Check sheet for the modelled part. Datum: model origin and axes. Units: mm. A direction names the side the tool comes from. Coordinates: 2 decimals unless noted, no trailing zeros. Loops run counter-clockwise (first coordinate to the right, second up) from the corner with the lowest first, then second, coordinate; pieces in that order, holes last.
Autodesk Inventor part; units mm, degrees
ref_plane "YZ Plane" through (0, 0, 0) normal (1, 0, 0) x (0, 1, 0)
ref_plane "XZ Plane" through (0, 0, 0) normal (0, 1, 0) x (-1, 0, 0)
ref_plane "XY Plane" through (0, 0, 0) normal (0, 0, 1) x (1, 0, 0)
sketch "Sketch6" plane through (0, 0, 0) normal (0, 1, 0) x (-1, 0, 0)
  line L0 (4.5, -6.1) -> (60.5, -6.1)
  line L1 (60.5, -6.1) -> (60.5, -90.9)
  line L2 (4.5, -90.9) -> (4.5, -6.1)
  line L3 (65.1201, -97) -> (0, -97)
  line L4 (0, -97) -> (0, 0)
  line L5 (0, 0) -> (65.1201, 0)
  line L6 (65.1201, 0) -> (65.1201, -97)
  line L7 (60.5, -90.9) -> (4.5, -90.9)
  line L8 (102.5, -48.5) -> (-37.5, -48.5)
  line L9 (32.5, -118.5) -> (32.5, 21.5)
  circle A0 centre (32.5, -48.5) radius 70
  line L10 (102.5, -48.5) -> (67.5, -109.1218)
  line L11 (67.5, -109.1218) -> (-2.5, -109.1218)
  line L12 (-2.5, -109.1218) -> (-37.5, -48.5)
  line L13 (-37.5, -48.5) -> (-2.5, 12.1218)
  line L14 (-2.5, 12.1218) -> (67.5, 12.1218)
  line L15 (67.5, 12.1218) -> (102.5, -48.5)
  line L16 (32.5, 12.1218) -> (85, -18.1891)
  line L17 (85, -18.1891) -> (85, -78.8109)
  line L18 (85, -78.8109) -> (32.5, -109.1218)
  line L19 (32.5, -109.1218) -> (-20, -78.8109)
  line L20 (-20, -78.8109) -> (-20, -18.1891)
  line L21 (-20, -18.1891) -> (32.5, 12.1218)
  line L22 (32.5, 12.1218) -> (47.5, 12.1218)
  line L23 (47.5, 12.1218) -> (47.5, 5.6218)
  line L24 (47.5, 5.6218) -> (17.5, 5.6218)
  line L25 (17.5, 5.6218) -> (17.5, 12.1218)
  line L26 (47.5, 5.6218) -> (56.6924, 5.6218) construction
  line L27 (17.5, 8.8718) -> (20, 8.8718)
  line L28 (47.5, 8.8718) -> (45, 8.8718)
  line L29 (45, 8.8718) -> (45, 10.1218)
  line L30 (45, 10.1218) -> (20, 10.1218)
  line L31 (20, 10.1218) -> (20, 7.6218)
  line L32 (20, 7.6218) -> (45, 7.6218)
  line L33 (45, 7.6218) -> (45, 10.1218)
  line L34 (67.5, 12.1218) -> (32.5, -48.5)
  line L35 (32.5, -48.5) -> (67.5, -109.1218)
  line L36 (47.5, 5.6218) -> (56.6924, 5.6218)
  line L37 (17.5, 5.6218) -> (11, 5.6218)
  line L38 (17.5, 12.1218) -> (11, 5.6218)
  line L39 (17.5, 12.1218) -> (26.6924, 12.1218) construction
  line L40 (47.5, 12.1218) -> (54, 5.6218)
  line L41 (85, -18.1891) -> (77.5, -5.1987)
  line L42 (77.5, -5.1987) -> (71.8708, -8.4487)
  line L43 (71.8708, -8.4487) -> (86.8708, -34.4295)
  line L44 (86.8708, -34.4295) -> (92.5, -31.1795)
  line L45 (71.8708, -8.4487) -> (67.2746, -0.4879) construction
  line L46 (89.6854, -32.8045) -> (88.4354, -30.6394)
  line L47 (74.6854, -6.8237) -> (75.9354, -8.9888)
  line L48 (75.9354, -8.9888) -> (77.0179, -8.3638)
  line L49 (77.0179, -8.3638) -> (89.5179, -30.0144)
  line L50 (89.5179, -30.0144) -> (87.3529, -31.2644)
  line L51 (87.3529, -31.2644) -> (74.8529, -9.6138)
  line L52 (74.8529, -9.6138) -> (77.0179, -8.3638)
  line L53 (71.8708, -8.4487) -> (67.2746, -0.4879)
  line L54 (86.8708, -34.4295) -> (90.1208, -40.0587)
  line L55 (92.5, -31.1795) -> (90.1208, -40.0587)
  line L56 (92.5, -31.1795) -> (87.9038, -23.2187) construction
  line L57 (77.5, -5.1987) -> (68.6208, -2.8196)
  line L58 (71.8708, -88.5513) -> (67.2746, -96.5121) construction
  line L59 (74.6854, -90.1763) -> (75.9354, -88.0112)
  line L60 (74.8529, -87.3862) -> (77.0179, -88.6362)
  line L61 (77.5, -91.8013) -> (71.8708, -88.5513)
  line L62 (77.5, -91.8013) -> (68.6208, -94.1804)
  line L63 (71.8708, -88.5513) -> (67.2746, -96.5121)
  line L64 (77.0179, -88.6362) -> (89.5179, -66.9856)
  line L65 (87.3529, -65.7356) -> (74.8529, -87.3862)
  line L66 (71.8708, -88.5513) -> (86.8708, -62.5705)
  line L67 (89.5179, -66.9856) -> (87.3529, -65.7356)
  line L68 (89.6854, -64.1955) -> (88.4354, -66.3606)
  line L69 (86.8708, -62.5705) -> (92.5, -65.8205)
  line L70 (86.8708, -62.5705) -> (90.1208, -56.9413)
  line L71 (92.5, -65.8205) -> (90.1208, -56.9413)
  line L72 (94.9944, -48.5) -> (63.7472, -102.6218)
  line L73 (63.7472, -102.6218) -> (1.2528, -102.6218)
  line L74 (1.2528, -102.6218) -> (-29.9944, -48.5)
  line L75 (-29.9944, -48.5) -> (1.2528, 5.6218)
  line L76 (1.2528, 5.6218) -> (63.7472, 5.6218)
  line L77 (63.7472, 5.6218) -> (94.9944, -48.5)
  line L78 (74.8529, -87.3862) -> (73.1208, -86.3862)
  line L79 (87.3529, -65.7356) -> (85.6208, -64.7356)
  line L80 (87.3529, -31.2644) -> (85.6208, -32.2644)
  line L81 (74.8529, -9.6138) -> (73.1208, -10.6138)
  line L82 (45, 7.6218) -> (45, 5.6218)
  line L83 (20, 7.6218) -> (20, 5.6218)
  line L84 (60.5, -90.9) -> (4.4985, -90.9)
  line L85 (4.4985, -90.9) -> (4.4985, -97)
  line L86 (4.4985, -97) -> (60.5, -97)
  line L87 (60.5, -97) -> (60.5, -90.9)
  line L88 (60.5, -6.1) -> (4.4985, -6.1)
  line L89 (4.4985, -6.1) -> (4.4985, 0)
  line L90 (4.4985, 0) -> (60.5, 0)
  line L91 (60.5, 0) -> (60.5, -6.1)
  dimension "d44" = 97
  dimension "d77" = 140
  dimension "d87" = 15
  dimension "d88" = 6.5
  dimension "d89" = 30
  dimension "d91" = 2.5
  dimension "d92" = 2.5
  dimension "d95" = 1.25
  dimension "d96" = 25
  dimension "d97" = 2.5
  dimension "d98" = 25
  dimension "d99" = 135
  dimension "d100" = 0
extrude "Fronte" add sketch "Sketch6" along normal blind 2 contours L89 L21 L5 L9 L0 | L2 L8 L4 L21 L89 | L9 L5 L16 L34 L0 | L2 L85 L19 L4 L8 | L89 L5 L21 | L21 L4 L5 L89 | L34 L16 L91 L0 | L9 L24 L16 L5 | L5 L21 L24 L9 | L7 L9 L3 L19 L85 | L8 L20 L75 L21 L4 | L4 L19 L74 L20 L8 | L21 L75 L76 L37 L24 L5 L4 | L91 L16 L6 L8 L1 | L34 L91 L16 | L16 L5 L34 | L8 L6 L18 L87 L1 | L7 L35 L18 L3 L9 | L7 L87 L18 L35 | L16 L24 L36 L76 L34 L5 | L24 L21 L32 L9 | L9 L32 L16 L24 | L85 L3 L4 L19 | L19 L3 L85 | L4 L3 L19 L73 L74 | L20 L74 L8 | L8 L75 L20 | L75 L20 L21 | L21 L13 L14 L38 L76 L75 | L24 L83 L32 L21 | L91 L5 L6 L16 | L34 L77 L53 L43 L16 L6 L5 | L8 L17 L66 L18 L6 | L6 L16 L43 L17 L8 | L9 L73 L19 L3 | L3 L18 L73 L9 | L35 L3 L18 | L18 L87 L35 | L16 L32 L82 L24 | L32 L21 L30 L9 | L9 L30 L16 L32 | L74 L73 L19 L11 L12 | L19 L20 L74 | L74 L20 L12 L8 | L8 L13 L20 L75 | L32 L31 L30 L21 | L24 L25 L27 L31 L83 | L76 L36 L40 L14 L34 | L34 L15 L57 L53 L77 | L18 L6 L3 L87 | L18 L66 L63 L72 L35 L3 L6 | L17 L43 L54 L77 L8 | L8 L72 L70 L66 L17 | L3 L35 L73 L18 | L73 L18 L9 | L9 L19 L73 | L16 L30 L29 L33 L32 | L82 L33 L28 L23 L24 | L30 L21 L9 | L9 L16 L30 | L38 L25 L37 | L30 L31 L27 L25 L14 L21 | L43 L81 L51 L16 | L16 L51 L17 L43 | L66 L17 L65 L18 | L18 L65 L78 L66 | L77 L55 L15 L8 | L8 L10 L71 L72 | L17 L51 L80 L43 | L66 L79 L65 L17 | L73 L35 L11 L18 | L72 L63 L62 L10 L35 | L16 L14 L23 L28 L29 L30 | L23 L40 L36 | L51 L52 L48 L49 L16 | L16 L49 L17 L51 | L43 L42 L47 L52 L81 | L15 L16 L49 L48 L47 L42 | L42 L53 L57 | L65 L17 L64 L18 | L18 L64 L60 L65 | L78 L60 L59 L61 L66 | L71 L69 L70 | L54 L44 L55 | L17 L49 L50 L51 | L80 L50 L46 L44 L43 | L65 L67 L64 L17 | L66 L69 L68 L67 L79 | L16 L17 L49 | L10 L17 L64 L67 L68 L69 | L44 L46 L50 L49 L17 L15 | L64 L17 L18 | L18 L10 L61 L59 L60 L64 | L61 L62 L63
extrude "Esterno" add sketch "Sketch6" against normal blind 25 contours L75 L20 L21 | L21 L13 L14 L38 L76 L75 | L74 L73 L19 L11 L12 | L19 L20 L74 | L74 L20 L12 L8 | L8 L13 L20 L75 | L76 L36 L40 L14 L34 | L34 L15 L57 L53 L77 | L73 L18 L9 | L9 L19 L73 | L77 L55 L15 L8 | L8 L10 L71 L72 | L73 L35 L11 L18 | L72 L63 L62 L10 L35
extrude "Strip" add sketch "Sketch6" against normal blind 10 contours L24 L21 L32 L9 | L9 L32 L16 L24 | L24 L83 L32 L21 | L16 L32 L82 L24 | L24 L25 L27 L31 L83 | L82 L33 L28 L23 L24 | L30 L21 L9 | L9 L16 L30 | L38 L25 L37 | L30 L31 L27 L25 L14 L21 | L43 L81 L51 L16 | L16 L51 L17 L43 | L66 L17 L65 L18 | L18 L65 L78 L66 | L17 L51 L80 L43 | L66 L79 L65 L17 | L16 L14 L23 L28 L29 L30 | L23 L40 L36 | L43 L42 L47 L52 L81 | L15 L16 L49 L48 L47 L42 | L42 L53 L57 | L78 L60 L59 L61 L66 | L71 L69 L70 | L54 L44 L55 | L80 L50 L46 L44 L43 | L66 L69 L68 L67 L79 | L16 L17 L49 | L10 L17 L64 L67 L68 L69 | L44 L46 L50 L49 L17 L15 | L64 L17 L18 | L18 L10 L61 L59 L60 L64 | L61 L62 L63
sketch "Sketch7" plane through (0, -25, 0) normal (0, -1, 0) x (1, 0, 0)
  line L0 (-17.5, 12.1218) -> (-17.5, -109.1218)
  line L1 (-67.5, -109.1218) -> (2.5, -109.1218)
  line L2 (-47.5, 12.1218) -> (-67.5, 12.1218)
  line L3 (-47.5, 12.1218) -> (-47.5, -109.1218)
  line L4 (-77.5, -91.8013) -> (-67.5, -109.1218)
  line L5 (-77.5, -91.8013) -> (27.5, -31.1795)
  line L6 (2.5, 12.1218) -> (37.5, -48.5)
  line L7 (-92.5, -65.8205) -> (-90.1208, -56.9413)
  line L8 (-92.5, -65.8205) -> (12.5, -5.1987)
  line L9 (-77.5, -5.1987) -> (27.5, -65.8205)
  line L10 (37.5, -48.5) -> (2.5, -109.1218)
  line L11 (-92.5, -31.1795) -> (11.423, -93.6666)
  line L12 (27.5, -31.1795) -> (12.5, -5.1987)
  line L13 (27.5, -65.8205) -> (11.423, -93.6666)
  line L14 (-1.2528, -102.6218) -> (29.9944, -48.5)
  line L15 (5.8516, -90.3166) -> (21.8708, -62.5705)
  line L16 (-47.5, -109.1218) -> (-17.5, -109.1218)
  line L17 (-17.5, -109.1218) -> (-17.5, -102.6218)
  line L18 (-17.5, -102.6218) -> (-47.5, -102.6218)
  line L19 (-47.5, -102.6218) -> (-47.5, -109.1218)
  line L20 (5.5339, -9.2206) -> (17.5, -36.953)
  point P0 (0, 0)
  point P1 (6.9325, -8.4131)
  point P2 (21.9325, -34.3939)
extrude "Passacavi" cut sketch "Sketch7" against normal blind 3 contours L0 L1 L3 L18 | L14 L9 L10 L11 | L20 L8 L6 L5
extrude "ScavoStrip" cut sketch "Sketch6" against normal blind 5 contours L24 L21 L32 L9 | L9 L32 L16 L24 | L24 L83 L32 L21 | L16 L32 L82 L24 | L43 L81 L51 L16 | L16 L51 L17 L43 | L66 L17 L65 L18 | L18 L65 L78 L66 | L17 L51 L80 L43 | L66 L79 L65 L17
extrude "ScreenDis1" add sketch "Sketch6" against normal blind 1 contours L7 L9 L3 L19 L85 | L7 L35 L18 L3 L9 | L7 L87 L18 L35 | L19 L3 L85 | L35 L3 L18 | L18 L87 L35
extrude "ScreenDist1.8" add sketch "Sketch6" against normal blind 1.8 contours L89 L21 L5 L9 L0 | L9 L5 L16 L34 L0 | L89 L5 L21 | L34 L16 L91 L0 | L34 L91 L16 | L16 L5 L34
properties part number "Hexagone" material "Wood (Cherry)"
1) Section check B-B on z = -80. Enter the section's corners in (x, y).
Answer sheet:
outline: (-84.31, -10) - (-82, -10) - (-82, 0) - (-60.5, 0) - (-60.5, 2) - (-84.31, 2) - close; (-79.12, -10) - (-76.81, -10) - (-76.81, -5) - (-79.12, -5) - close; (-4.5, 0) - (11.81, 0) - (11.81, -22) - (19.31, -22) - (19.31, 2) - (-4.5, 2) - close
2) Depth check by flat-ended pin: pin 1 (1.8 mm diameter, centred on x = -45, z = -2, fed in from -Y); pin 2 (1.4 mm diameter, centred on y = -0.5, z = -2, fed in from -X); pin 3 (0.6 mm diameter, centred on y = 1.5, z = -33, fed in from +X). Enter the tip coordinate at first touch or a pass-through.
Answer sheet:
pin 1: stops at y = -1.8
pin 2: stops at x = -76.06
pin 3: stops at x = 28.72
3) Scan lines: line 1 (Z direction, x = -26, y = -7); line 2 (Z direction, x = -12.5, y = -6.25); line 3 (Z direction, x = -42, y = -2.75). Record each from-to range of solid material in increasing order.
Answer sheet:
line 1: z = -109.12 to -102.62, 5.62 to 7.62, 10.12 to 12.12
line 2: z = -109.12 to -102.62, 5.62 to 12.12
line 3: z = -109.12 to -102.62, 10.12 to 12.12
4) Section check C-C on x = -57. Enter the section's corners in (y, z).
Answer sheet:
outline: (-25, -109.12) - (2, -109.12) - (2, -90.9) - (-1, -90.9) - (-1, -97) - (0, -97) - (0, -102.62) - (-25, -102.62) - close; (-25, 5.62) - (0, 5.62) - (0, 0) - (-1.8, 0) - (-1.8, -6.1) - (2, -6.1) - (2, 12.12) - (-25, 12.12) - close
5) Section check D-D on z = -36. Enter the section's corners in (x, y), plus the area to 3 significant figures.
Answer sheet:
outline: (-95.28, -25) - (-91.21, -25) - (-91.21, -10) - (-87.78, -10) - (-87.78, 0) - (-60.5, 0) - (-60.5, 2) - (-95.28, 2) - close; (-4.5, 0) - (22.78, 0) - (22.78, -25) - (30.28, -25) - (30.28, 2) - (-4.5, 2) - close
area: 463 mm2
6) Mould release check, pull along Z, two halves, no side actions. Record for faces 1 (the flat face through (24.646, -23.521, -32.827)), 2 (the flat face through (-73.123, -17.395, -4.026)), 3 (the flat face through (-91.327, -17.395, -61.443)): +Z half, -Z half, draft (parallel to the pull), parting line (faces both ways), or undercut.
Answer sheet:
face 1: +Z half
face 2: undercut
face 3: -Z half
7) Set-up check for faces 4 (the flat face through (-33, -22, -106)), 5 (the flat face through (-32, 0, -6.1)), 6 (the flat face through (-80.5, -10, -20)): record each of +Z, -Z, +X, -X, +Y, -Y from which the full face is reachable in a straight line by a thin tool's end or side.
Answer sheet:
face 4: +Z, -Z, -Y
face 5: +Y, -Y
face 6: -Y
8) Section check A-A on x = -27. Enter the section's corners in (y, z).
Answer sheet:
outline: (-22, -109.12) - (2, -109.12) - (2, -90.9) - (-1, -90.9) - (-1, -97) - (0, -97) - (0, -102.62) - (-22, -102.62) - close; (-10, 5.62) - (-5, 5.62) - (-5, 7.62) - (-10, 7.62) - close; (-10, 10.12) - (0, 10.12) - (0, 0) - (-1.8, 0) - (-1.8, -6.1) - (2, -6.1) - (2, 12.12) - (-10, 12.12) - close
